from build123d import *
from build123d import SkipClean  # not in build123d's __all__

# Parameters (mm, degrees)
F0_R     = 10.16
F1_DEPTH = 15.7734
F3_DEPTH = 24.4602
F4_R     = 3.302


with BuildPart() as f1:
    # F0 (on Top) → F1 (new body)
    with BuildSketch(Plane.XY):
        with BuildLine():
            Line((5.865458004, 27.9665340613), (4.2022058824, 28.2643254072))
            ThreePointArc((4.2022058824, 28.2643254072), (-28.575, 0), (4.2022058824, -28.2643254072))
            Line((4.2022058824, -28.2643254072), (5.865458004, -27.9665340613))
            ThreePointArc((5.865458004, -27.9665340613), (22.182606784, -18.0128448966), (28.575, 0))
            ThreePointArc((28.575, 0), (22.182606784, 18.0128448966), (5.865458004, 27.9665340613))
        make_face()
        with BuildLine():
            ThreePointArc((13.4477648793, -4.826), (-14.2875, 0), (13.4477648793, 4.826))
            Line((13.4477648793, 4.826), (18.5293, 4.826))
            Line((18.5293, 4.826), (18.5293, -4.826))
            Line((18.5293, -4.826), (13.4477648793, -4.826))
        make_face(mode=Mode.SUBTRACT)
        with BuildLine():
            ThreePointArc((5.865458004, 27.9665340613), (5.0360335537, 28.1277263753), (4.2022058824, 28.2643254072))
            Line((4.2022058824, 28.2643254072), (5.865458004, 27.9665340613))
        make_face()
        with BuildLine():
            Line((5.865458004, -27.9665340613), (4.2022058824, -28.2643254072))
            ThreePointArc((4.2022058824, -28.2643254072), (5.0360335537, -28.1277263753), (5.865458004, -27.9665340613))
        make_face()
        with BuildLine():
            Line((57.3323557024, 18.7518175836), (5.865458004, 27.9665340613))
            ThreePointArc((5.865458004, 27.9665340613), (22.182606784, 18.0128448966), (28.575, 0))
            ThreePointArc((28.575, 0), (22.182606784, -18.0128448966), (5.865458004, -27.9665340613))
            Line((5.865458004, -27.9665340613), (57.3323557024, -18.7518175836))
            ThreePointArc((57.3323557024, -18.7518175836), (34.925, 0), (57.3323557024, 18.7518175836))
        make_face()
        with BuildLine():
            ThreePointArc((73.025, 0), (68.5842458076, 12.2258920711), (57.3323557024, 18.7518175836))
            ThreePointArc((57.3323557024, 18.7518175836), (34.925, 0), (57.3323557024, -18.7518175836))
            ThreePointArc((57.3323557024, -18.7518175836), (68.5842458076, -12.2258920711), (73.025, 0))
        make_face()
        with Locations((53.975, 0)):
            Circle(F0_R, mode=Mode.SUBTRACT)
    extrude(amount=-F1_DEPTH)

    # F2 (on face) → F3 (join)
    with BuildSketch(Plane.XY):
        with BuildLine():
            ThreePointArc((28.575, 0), (22.182606784, 18.0128448966), (5.865458004, 27.9665340613))
            ThreePointArc((5.865458004, 27.9665340613), (-28.575, 0), (5.865458004, -27.9665340613))
            ThreePointArc((5.865458004, -27.9665340613), (22.182606784, -18.0128448966), (28.575, 0))
        make_face()
        with BuildLine():
            ThreePointArc((13.4477648793, -4.826), (-14.2875, 0), (13.4477648793, 4.826))
            Line((13.4477648793, 4.826), (18.5293, 4.826))
            Line((18.5293, 4.826), (18.5293, -4.826))
            Line((18.5293, -4.826), (13.4477648793, -4.826))
        make_face(mode=Mode.SUBTRACT)
    with SkipClean():  # cleaning this boolean's faces spoils the solid; the shape is the same uncleaned
        extrude(amount=F3_DEPTH)

    # F4
    f4_edges = [f1.edges().sort_by_distance(p)[0] for p in [
        (-5.865458, 27.966534, 24.4602),
    ]]
    fillet(f4_edges, radius=F4_R)


solid = f1.part
The model under review builds one solid part; all positions refer to its coordinate system, in mm. A direction names the side the tool comes from. Give positions to 0.01 mm unless a question says otherwise; leave off trailing zeros.
1. Draft analysis for pull direction Y (two halves, no side actions). For faces 3 (the flat face through (39, 0, 0)), 4 (the flat face through (31.239, -23.424, -7.776)), 5 (the flat face through (31.959, 23.295, -7.776)), 6 (the cylindrical face through (43.825, 0.447, -7.776)), state which applies: +Y half, -Y half, draft (parallel to the pull), parting line (faces both ways), or undercut.
2. Wall thickness on L1, parallel to Y at x = 0, z = 13 (1 decimal); L2, parallel to X at y = 3.5, z = -4; L3, parallel to Z at x = 63, y = 8.5: over which ranges is each line inside the solid? List them lowest first.
3. For P1, Ø1.5, axis at x = 15.5, z = -4.5, coming from the -Y side; P2, Ø3, axis at x = 35.5, z = -8.5, coming from the -Y side; P3, Ø10, axis at y = 4.5, z = 17.5, coming from the +X side (3 decimals), all flat-tipped, find the tip position at first contact; note any pin that passes through.
4. Add section B-B, the plane z = -1. Count the separate pieces of the cut face and the enclosed holes in it, plus the area to 3 significant figures.
5. Tool access review of faces 1 (the flat face through (11, -11, 24.46)), 2 (the flat face through (16, 4.826, 4)): name each direction out of +Z, -Z, +X, -X, +Y, -Y from which nothing blocks a thin tool from reaching the whole face with its end or side.
Worked answers:
1. face 3: draft
1. face 4: -Y half
1. face 5: +Y half
1. face 6: undercut
2. L1: y = -28.6 to -14.3, 14.3 to 28.6
2. L2: x = -28.36 to -13.85, 18.53 to 44.44, 63.51 to 72.7
2. L3: z = -15.77 to 0
3. P1: stops at y = -26.38
3. P2: stops at y = -22.93
3. P3: stops at x = 28.575
4. separate pieces: 1
4. enclosed holes: 2
4. area: 3,450 mm2
5. face 1: +Z, +X, -X, +Y, -Y
5. face 2: +Z, -Z
